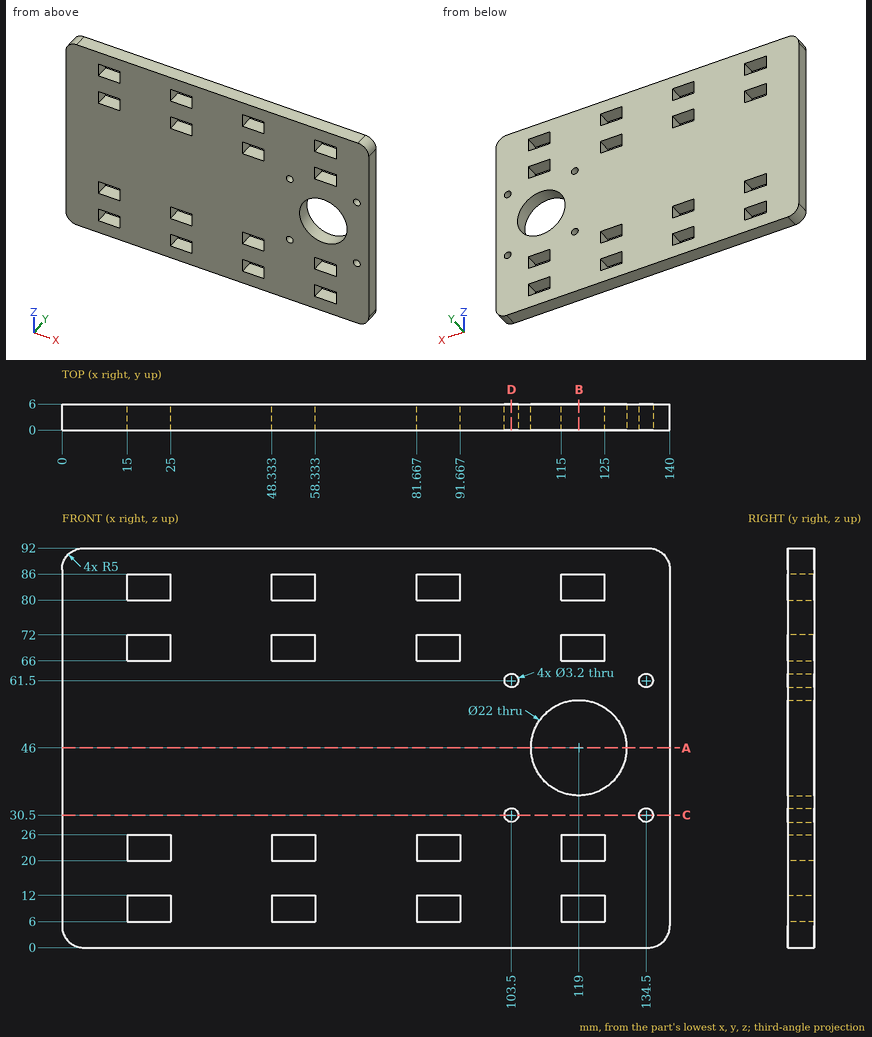
Could you check a few things on this drawing? It's one solid part, dimensions in mm from its lowest x, y, z. Round coordinates to 2 decimals unless told otherwise and drop trailing zeros. Write each loop counter-clockwise with the first axis right and the second up, starting at its lowest first coordinate (ties: lowest second). Pieces come first, ordered by that corner, then holes.
Q1. Will this pin go through, and if not, where does the flat tip stop? P1, Ø1.8, axis at x = 18.5, y = 4.5, coming from the -Z side.
Q2. If we section it at B-B on x = 119: Write out the boundary of the cut face in (y, z).
Q3. Please list where these lines run through material, in increasing order: probe 1 along Z at (x, y) = (103.5, 1.3); probe 2 along Z at (x, y) = (55, 1.4); probe 3 along Z at (x, y) = (119, 3.55).
Q4. If we section it at A-A on z = 46: Write out the boundary of the cut face in (x, y).
Q5. If we section it at D-D on x = 103.5: Write out the boundary of the cut face in (y, z).
Q6. If we section it at C-C on z = 30.5: Write out the boundary of the cut face in (x, y).
Answer below:
1. P1: stops at z = 0
2. outline: (0, 0) - (6, 0) - (6, 6) - (0, 6) - close; (0, 12) - (6, 12) - (6, 20) - (0, 20) - close; (0, 26) - (6, 26) - (6, 35) - (0, 35) - close; (0, 57) - (6, 57) - (6, 66) - (0, 66) - close; (0, 72) - (6, 72) - (6, 80) - (0, 80) - close; (0, 86) - (6, 86) - (6, 92) - (0, 92) - close
3. probe 1: z = 0 to 28.9, 32.1 to 59.9, 63.1 to 92
3. probe 2: z = 0 to 6, 12 to 20, 26 to 66, 72 to 80, 86 to 92
3. probe 3: z = 0 to 6, 12 to 20, 26 to 35, 57 to 66, 72 to 80, 86 to 92
4. outline: (0, 0) - (108, 0) - (108, 6) - (0, 6) - close; (130, 0) - (140, 0) - (140, 6) - (130, 6) - close
5. outline: (0, 0) - (6, 0) - (6, 28.9) - (0, 28.9) - close; (0, 32.1) - (6, 32.1) - (6, 59.9) - (0, 59.9) - close; (0, 63.1) - (6, 63.1) - (6, 92) - (0, 92) - close
6. outline: (0, 0) - (101.9, 0) - (101.9, 6) - (0, 6) - close; (105.1, 0) - (132.9, 0) - (132.9, 6) - (105.1, 6) - close; (136.1, 0) - (140, 0) - (140, 6) - (136.1, 6) - close
